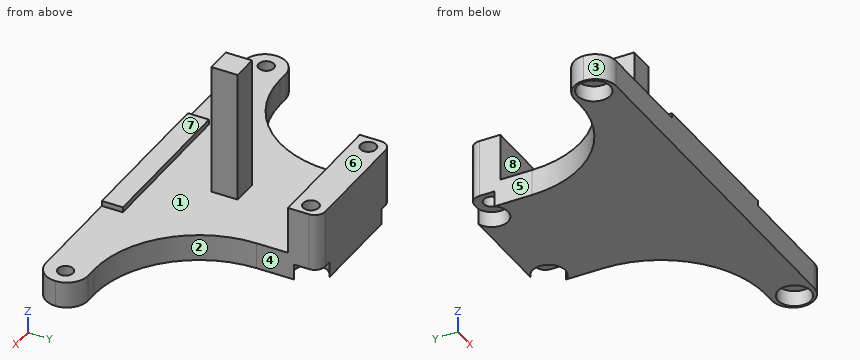
```python
from build123d import *

# Parameters (mm, degrees)
SKETCH_1_W          = 77
SKETCH_1_H          = 8
SKETCH_1_R          = 1.45
EXTRUDE_1_DEPTH     = 5
SKETCH_2_W          = 25
SKETCH_2_H          = 32
SKETCH_2_R          = 1.5
EXTRUDE_2_DEPTH     = 5
SKETCH_3_W          = 25
SKETCH_3_H          = 6
SKETCH_3_R          = 1.5
EXTRUDE_3_DEPTH     = 9
FILLET_1_R          = 20
FILLET_2_R          = 4
FILLET_3_R          = 2
SKETCH_4_R          = 3.125
CUT_EXTRUDE_3_DEPTH = 3
SKETCH_5_W          = 30
SKETCH_5_H          = 4
EXTRUDE_4_DEPTH     = 1
SKETCH_6_W          = 5
SKETCH_6_H          = 5
EXTRUDE_5_DEPTH     = 25


with BuildPart() as part:
    # Эскиз1 → Бобышка-Вытянуть1 (new body)
    with BuildSketch(Plane.XY):
        Rectangle(SKETCH_1_W, SKETCH_1_H)
        with Locations((-35, 0)):
            Circle(SKETCH_1_R, mode=Mode.SUBTRACT)
        with Locations((35, 0)):
            Circle(SKETCH_1_R, mode=Mode.SUBTRACT)
    extrude(amount=EXTRUDE_1_DEPTH)

    # Эскиз2 → Бобышка-Вытянуть2 (add)
    with BuildSketch(Plane(origin=(0, 0, 0), x_dir=(-1, 0, 0), z_dir=(0, 0, -1))):
        with Locations((0, 20)):
            Rectangle(SKETCH_2_W, SKETCH_2_H)
        with Locations((-10, 33)):
            Circle(SKETCH_2_R, mode=Mode.SUBTRACT)
        with Locations((10, 33)):
            Circle(SKETCH_2_R, mode=Mode.SUBTRACT)
    extrude(amount=-EXTRUDE_2_DEPTH)

    # Эскиз3 → Бобышка-Вытянуть3 (add)
    with BuildSketch(Plane(origin=(0, 0, 5), x_dir=(-1, 0, 0), z_dir=(0, 0, -1))):
        with Locations((0, 33)):
            Rectangle(SKETCH_3_W, SKETCH_3_H)
        with Locations((10, 33)):
            Circle(SKETCH_3_R, mode=Mode.SUBTRACT)
        with Locations((-10, 33)):
            Circle(SKETCH_3_R, mode=Mode.SUBTRACT)
    extrude(amount=-EXTRUDE_3_DEPTH)

    # Скругление1
    fillet_1_edges = [part.edges().sort_by_distance(p)[0] for p in [
        (12.5, 4, 2.5),
        (-12.5, 4, 2.5),
    ]]
    fillet(fillet_1_edges, radius=FILLET_1_R)

    # Скругление2
    fillet_2_edges = [part.edges().sort_by_distance(p)[0] for p in [
        (-38.5, -4, 2.5),
        (-38.5, 4, 2.5),
        (38.5, -4, 2.5),
        (38.5, 4, 2.5),
    ]]
    fillet(fillet_2_edges, radius=FILLET_2_R - 0.0001)  # a hair under: the kernel refuses the full size

    # Скругление3
    fillet_3_edges = [part.edges().sort_by_distance(p)[0] for p in [
        (12.5, 36, 7),
        (-12.5, 36, 7),
    ]]
    fillet(fillet_3_edges, radius=FILLET_3_R)

    # Эскиз4 → Вырез-Вытянуть3 (cut)
    with BuildSketch(Plane(origin=(0, 0, 0), x_dir=(-1, 0, 0), z_dir=(0, 0, -1))):
        with Locations((-10, 33)):
            Circle(SKETCH_4_R)
        with Locations((10, 33)):
            Circle(SKETCH_4_R)
        with Locations((-35, 0)):
            Circle(SKETCH_4_R)
        with Locations((35, 0)):
            Circle(SKETCH_4_R)
    extrude(amount=-CUT_EXTRUDE_3_DEPTH, mode=Mode.SUBTRACT)

    # Эскиз5 → Бобышка-Вытянуть4 (add)
    with BuildSketch(Plane.XY.offset(5)):
        with Locations((0, -2)):
            Rectangle(SKETCH_5_W, SKETCH_5_H)
    extrude(amount=EXTRUDE_4_DEPTH)

    # Эскиз6 → Бобышка-Вытянуть5 (add)
    with BuildSketch(Plane.XY.offset(5)):
        with Locations((0, 12.5)):
            Rectangle(SKETCH_6_W, SKETCH_6_H)
    extrude(amount=EXTRUDE_5_DEPTH)


solid = part.part
```
Here's how the part is built. I have some questions about the finished solid (model axes, mm). Face numbers are marked on the shaded views. A direction names the side the tool comes from. Coordinates: 2 decimals unless noted, no trailing zeros. Write each loop counter-clockwise with the first axis right and the second up, starting at its lowest first coordinate (ties: lowest second). Pieces come first, ordered by that corner, then holes. Notation, with made-up numbers: (11.5, 13.5) - (60.5, 13.5) arc R26 ccw to (60.5, 49.5) - close; hole circle Ø5 at (-29, -7.5). An arc over 180 degrees is marked (long way). One line per item, written item: value.
1) Suppose I cut it at A-A on z = 12.5. Write out the boundary of the cut face in (x, y), and give its area (3 significant figures).
Model answer:
outline: (-12.5, 30) - (12.5, 30) - (12.5, 34) arc R2 ccw to (10.5, 36) - (-10.5, 36) arc R2 ccw to (-12.5, 34) - close; (-2.5, 10) - (2.5, 10) - (2.5, 15) - (-2.5, 15) - close; hole circle Ø3 at (-10, 33); hole circle Ø3 at (10, 33)
area: 159 mm²
2) On a 3-axis mill with a long thin cutter (end or side, diameter ignored), from which of +Z, -Z, +X, -X, +Y, -Y can I reach the whole of each face in a straight line? I mean the marked faces 4, 5, 6, 7 and 8. Say none if no direction works.
Model answer:
face 4: +Z, -Z, +X, +Y
face 5: +Z, -Z, -X, +Y
face 6: +Z, +X, -X, +Y
face 7: +Z, +X, -X, -Y
face 8: +Z, +X, -X
3) I'm going to push flat-ended pins straight in: P1, Ø5, axis at y = 29.5, z = 7, coming from the -X side; P2, Ø1.6, axis at x = -33.5, z = 3, coming from the +Y side; P3, Ø5.5, axis at x = -35, y = 0, coming from the -Z side. Where does each tip first touch, or does it pass through?
Model answer:
P1: stops at x = -12.5
P2: stops at y = 4
P3: stops at z = 3
4) Suppose I cut it at B-B on x = -5.5. Write out the boundary of the cut face in (y, z), and give its area (3 significant figures).
Model answer:
outline: (-4, 0) - (36, 0) - (36, 14) - (30, 14) - (30, 5) - (0, 5) - (0, 6) - (-4, 6) - close
area: 258 mm²
5) I need wall thicknesses on line 1 along Y through (x, z) = (10, 8.25); line 2 along Z through (x, y) = (2, -0.5); line 3 along X through (y, z) = (25.5, 2.25). Which ranges of each line are inside material? Lowest first, please.
Model answer:
line 1: y = 30 to 31.5, 34.5 to 36
line 2: z = 0 to 6
line 3: x = -12.5 to 12.5
6) We'd pull the mould along Y, two halves only. Please class the marked faces 1, 2 and 3: pulls with the +Y half, pulls with the -Y half, needs draft (parallel to the pull), parting line crosses it, or undercut.
Model answer:
face 1: undercut
face 2: pulls with the +Y half
face 3: pulls with the -Y half
7) Suppose I cut it at C-C on y = 8. Write out the boundary of the cut face in (x, z).
Model answer:
outline: (-20.5, 0) - (20.5, 0) - (20.5, 5) - (-20.5, 5) - close
8) Suppose I cut it at D-D on z = 2. State how many separate pieces and enclosed holes the cut face has, and give its area (3 significant figures).
Model answer:
separate pieces: 1
enclosed holes: 2
area: 1,450 mm²
